```python
from build123d import *

# Parameters (mm, degrees)
SKETCH1_W                           = 139.7
SKETCH1_H                           = 127
SKETCH1_R                           = 4.7625
BOSS_EXTRUDE1_DEPTH                 = 12
TAP_DRILL_FOR_10_24_TAP1_AT_2_COUNT = 2
TAP_DRILL_FOR_10_24_TAP1_AT_2_PITCH = 50.8
TAP_DRILL_FOR_10_24_TAP1_AT_3_COUNT = 2
TAP_DRILL_FOR_10_24_TAP1_AT_3_PITCH = 101.6


with BuildPart() as part:
    # Sketch1 → Boss-Extrude1 (new body)
    with BuildSketch(Plane.XY):
        with Locations((0, 12.7)):
            Rectangle(SKETCH1_W, SKETCH1_H)
        with Locations((0, 14.67)):
            Circle(SKETCH1_R, mode=Mode.SUBTRACT)
    extrude(amount=BOSS_EXTRUDE1_DEPTH)

    # Sketch4 → Tap Drill for #10-24 Tap1 (revolve, cut)
    with BuildSketch(Plane(origin=(50.8, -50.8, 6), x_dir=(0, 0, -1), z_dir=(1, 0, 0))):
        Polygon((0, 0), (0, 13.840824014), (1.89865, 12.7), (1.89865, 0), align=None)
    tap_drill_for_10_24_tap1 = revolve(axis=Axis((50.8, -57.15, 6), (0, 1, 0)), mode=Mode.SUBTRACT)

    # Tap Drill for #10-24 Tap1 at 2: Tap Drill for #10-24 Tap1 ×2
    with Locations(*[(-i * TAP_DRILL_FOR_10_24_TAP1_AT_2_PITCH, 0, 0) for i in range(1, TAP_DRILL_FOR_10_24_TAP1_AT_2_COUNT)]):
        add(tap_drill_for_10_24_tap1, mode=Mode.SUBTRACT)

    # Tap Drill for #10-24 Tap1 at 3: Tap Drill for #10-24 Tap1 ×2
    with Locations(*[(-i * TAP_DRILL_FOR_10_24_TAP1_AT_3_PITCH, 0, 0) for i in range(1, TAP_DRILL_FOR_10_24_TAP1_AT_3_COUNT)]):
        add(tap_drill_for_10_24_tap1, mode=Mode.SUBTRACT)

    # Mirror1: Tap Drill for #10-24 Tap1 across plane
    add(tap_drill_for_10_24_tap1.mirror(Plane(origin=(0, 12.7, 0), x_dir=(0, 0, 1), z_dir=(0, -1, 0))), mode=Mode.SUBTRACT)

    # Mirror1 copy 1 sketch → Mirror1 copy 1 (revolve, cut)
    with BuildSketch(Plane(origin=(0, 76.2, 6), x_dir=(0, 0, -1), z_dir=(1, 0, 0))):
        Polygon((0, 0), (0, -13.840824014), (1.89865, -12.7), (1.89865, 0), align=None)
    revolve(axis=Axis((0, 82.55, 6), (0, 1, 0)), mode=Mode.SUBTRACT)

    # Mirror1 copy 2 sketch → Mirror1 copy 2 (revolve, cut)
    with BuildSketch(Plane(origin=(-50.8, 76.2, 6), x_dir=(0, 0, -1), z_dir=(1, 0, 0))):
        Polygon((0, 0), (0, -13.840824014), (1.89865, -12.7), (1.89865, 0), align=None)
    revolve(axis=Axis((-50.8, 82.55, 6), (0, 1, 0)), mode=Mode.SUBTRACT)


solid = part.part
```
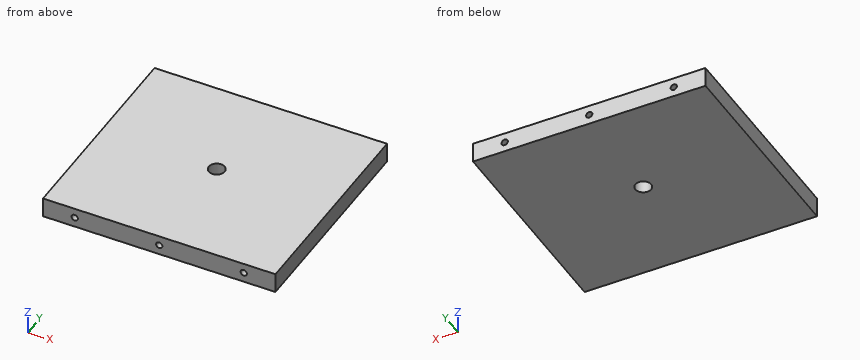
Read the model definition and answer for the solid it produces. Units are mm, in the model's axes. Give positions to 0.01 mm unless a question says otherwise; leave off trailing zeros. Order: outer loops, then holes, each group sorted by start corner. A loop starts at its lowest first (then second) coordinate and runs counter-clockwise, first axis right, second up. Notation, with made-up numbers: (-30, 47) -> (2, 47) arc R22 ccw to (2, 61) -> close; hole circle Ø3 at (9, 42). An arc over 180 degrees is marked (long way). One line per item, written item: value. Start each with the question number.
(1) Straight lines are drawn through the part: L1, parallel to X at y = -44.75, z = 6; L2, parallel to Z at x = -50.8, y = 70; L3, parallel to Y at x = 0, z = 8.75. For each, find the intervals that lie inside material, in ascending order.
(2) Flat-ended cylindrical pins translate along their axes: P1, Ø4.5, axis at x = 0, z = 6, coming from the +Y side; P2, Ø2.5, axis at x = 50.8, z = 6, coming from the -Y side; P3, Ø3.5, axis at x = 0, z = 6, coming from the +Y side; P4, Ø3, axis at x = -50.8, z = 6, coming from the -Y side. Find the tip coordinate at first contact, or state that the pin passes through.
(3) The part is cut by section A-A (y = 14.67). Determine the outline of the cut face in (x, z).
Taken from the geometry:
1. L1: -69.85 to -52.7, -48.9 to -1.9, 1.9 to 48.9, 52.7 to 69.85
1. L2: 0 to 4.1, 7.9 to 12
1. L3: -50.8 to 9.91, 19.43 to 76.2
2. P1: y = 76.2
2. P2: y = -37.71
2. P3: y = 63.41
2. P4: y = -37.86
3. outline: (-69.85, 0) -> (-4.76, 0) -> (-4.76, 12) -> (-69.85, 12) -> close; (4.76, 0) -> (69.85, 0) -> (69.85, 12) -> (4.76, 12) -> close
